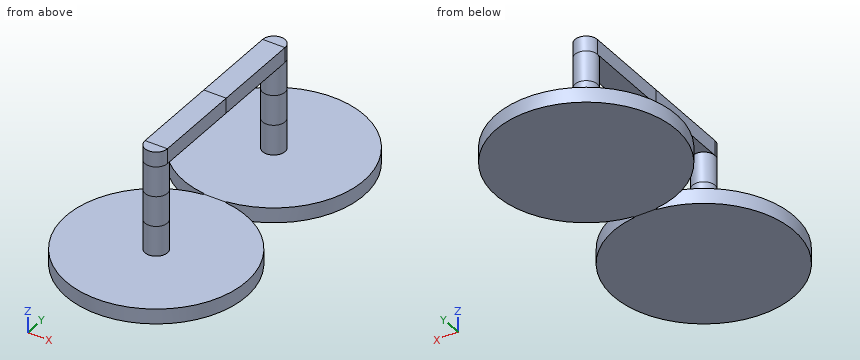
from build123d import *

# Parameters (mm, degrees)
SKETCH_1_R                       = 1.49
EXTRUDE_1_DEPTH                  = 4
EXTRUDE_START                    = 4
SKETCH_2_R                       = 1.49
EXTRUDE_2_DEPTH                  = 4
SKETCH_3_R                       = 1.49
EXTRUDE_3_DEPTH                  = 4
SKETCH_4_W                       = 2.98
SKETCH_4_H                       = 2
EXTRUDE_4_DEPTH                  = 12
EXTRUDE_4_DIRECTION_2_REACH      = 10.273
EXTRUDE_4_DIRECTION_2_END_RADIUS = 1.49
SKETCH_9_R                       = 12
EXTRUDE_6_DEPTH                  = 2
SKETCH_6_W                       = 2.98
SKETCH_6_H                       = 2
EXTRUDE_5_DEPTH                  = 12
EXTRUDE_5_DIRECTION_2_REACH      = 20.762
EXTRUDE_5_DIRECTION_2_END_RADIUS = 1.49


with BuildPart() as part:
    # 草图1 → 凸台-拉伸1 (new body)
    with BuildSketch(Plane.XY):
        Circle(SKETCH_1_R)
    extrude(amount=EXTRUDE_1_DEPTH)

    # 草图2 → 凸台-拉伸2 (add)
    with BuildSketch(Plane(origin=(0, 0, 0), x_dir=(-1, 0, 0), z_dir=(0, 0, -1)).offset(EXTRUDE_START)):
        Circle(SKETCH_2_R)
    extrude(amount=-EXTRUDE_2_DEPTH)

    # 草图3 → 凸台-拉伸3 (add)
    with BuildSketch(Plane.XY.offset(4)):
        with Locations(Location((0, 0, 0), (0, 0, 180))):
            Circle(SKETCH_3_R)
    extrude(amount=EXTRUDE_3_DEPTH)

    # 草图4 → 凸台-拉伸4 (add)
    with BuildSketch(Plane(origin=(0, 0, 0), x_dir=(1, 0, 0), z_dir=(0, 1, 0))):
        with Locations((0, 5)):
            Rectangle(SKETCH_4_W, SKETCH_4_H)
    extrude(amount=EXTRUDE_4_DEPTH)

    # 凸台-拉伸4 direction 2: up to this cylinder (the profile starts inside it)
    extrude_4_direction_2_end = Plane(origin=(0, 0, -5), z_dir=(0, 0, -1)) * Cylinder(EXTRUDE_4_DIRECTION_2_END_RADIUS, 24.526, mode=Mode.PRIVATE)
    # 草图4 → 凸台-拉伸4 direction 2 (add, up to the surface)
    with BuildSketch(Plane(origin=(0, 0, 0), x_dir=(1, 0, 0), z_dir=(0, 1, 0)), mode=Mode.PRIVATE) as extrude_4_direction_2_sk1:
        with Locations((0, 5)):
            Rectangle(SKETCH_4_W, SKETCH_4_H)
    extrude_4_direction_2_tool1 = extrude(extrude_4_direction_2_sk1.sketch, amount=-EXTRUDE_4_DIRECTION_2_REACH, mode=Mode.PRIVATE) & extrude_4_direction_2_end
    add(extrude_4_direction_2_tool1.solids().sort_by_distance((0, 0, -5))[0])

    # 草图9 → 凸台-拉伸6 (add)
    with BuildSketch(Plane(origin=(0, 0, -6), x_dir=(-1, 0, 0), z_dir=(0, 0, -1))):
        Circle(SKETCH_9_R)
    extrude(amount=-EXTRUDE_6_DEPTH)

    # 草图6 → 凸台-拉伸5 (add)
    with BuildSketch(Plane(origin=(0, 0, 0), x_dir=(1, 0, 0), z_dir=(0, 1, 0))):
        with Locations((0, -9)):
            Rectangle(SKETCH_6_W, SKETCH_6_H)
    extrude(amount=EXTRUDE_5_DEPTH)

    # 凸台-拉伸5 direction 2: up to this cylinder (the profile starts inside it)
    extrude_5_direction_2_end = Plane(origin=(0, 0, 9), z_dir=(0, 0, -1)) * Cylinder(EXTRUDE_5_DIRECTION_2_END_RADIUS, 45.504, mode=Mode.PRIVATE)
    # 草图6 → 凸台-拉伸5 direction 2 (add, up to the surface)
    with BuildSketch(Plane(origin=(0, 0, 0), x_dir=(1, 0, 0), z_dir=(0, 1, 0)), mode=Mode.PRIVATE) as extrude_5_direction_2_sk1:
        with Locations((0, -9)):
            Rectangle(SKETCH_6_W, SKETCH_6_H)
    extrude_5_direction_2_tool1 = extrude(extrude_5_direction_2_sk1.sketch, amount=-EXTRUDE_5_DIRECTION_2_REACH, mode=Mode.PRIVATE) & extrude_5_direction_2_end
    add(extrude_5_direction_2_tool1.solids().sort_by_distance((0, 0, 9))[0])

    # 镜向2: part across plane


with BuildPart() as part_1:
    add(part.part)
    add(part.part.mirror(Plane.ZX.offset(12)))


solid = part_1.part
The listing builds one solid part. Answer for the finished solid, in the listing's coordinates (mm). Coordinates: 2 decimals unless noted, no trailing zeros. Write each loop counter-clockwise with the first axis right and the second up, starting at its lowest first coordinate (ties: lowest second). Pieces come first, ordered by that corner, then holes. Notation, with made-up numbers: (19.5, 86) - (61.5, 86) arc R30 ccw to (61.5, 113) - close; hole circle Ø9 at (-11.5, 77). An arc over 180 degrees is marked (long way). Return JSON: item names as keys, results as strings.
1. The part is cut by section A-A on x = -3. Determine the outline of the cut face in (y, z).
Final values:
{"outline": "(-11.62, -6) - (11.62, -6) - (11.62, -4) - (-11.62, -4) - close; (12.38, -6) - (35.62, -6) - (35.62, -4) - (12.38, -4) - close"}
2. The part is cut by section B-B on y = 2.5. Determine the outline of the cut face in (x, z).
Final values:
{"outline": "(-11.74, -6) - (11.74, -6) - (11.74, -4) - (-11.74, -4) - close; (-1.49, 8) - (1.49, 8) - (1.49, 10) - (-1.49, 10) - close"}
3. The part is cut by section C-C on x = 0. Determine the outline of the cut face in (y, z), then the cut area to 3 significant figures.
Final values:
{"outline": "(-12, -6) - (36, -6) - (36, -4) - (25.49, -4) - (25.49, 10) - (-1.49, 10) - (-1.49, -4) - (-12, -4) - close; hole (1.49, -4) - (22.51, -4) - (22.51, 8) - (1.49, 8) - close", "area": "221 mm^2"}
4. Each of these flat-tipped pins is pushed along its axis until it touches: pin 1 Ø2 at (x, y) = (6.5, 24.5) entering from +Z; pin 2 Ø2 at (y, z) = (20.5, 9) entering from -X; pin 3 Ø0.6 at (y, z) = (15, 8.5) entering from +X. Where does it stop, or does it pass through?
Final values:
{"pin 1": "z = -4", "pin 2": "x = -1.49", "pin 3": "x = 1.49"}
5. Consider line 1 along Z through (x, y) = (-3.25, 14); line 2 along Y through (x, z) = (-7, -5); line 3 along Y through (x, z) = (-6, -4.5). Determine where each line is inside the solid, lowest interval first.
Final values:
{"line 1": "-6 to -4", "line 2": "-9.75 to 9.75, 14.25 to 33.75", "line 3": "-10.39 to 10.39, 13.61 to 34.39"}
6. The part is cut by section D-D on z = 2.5. Determine the outline of the cut face in (x, y), then the cut area to 3 significant figures.
Final values:
{"outline": "circle Ø2.98 at (0, 0); circle Ø2.98 at (0, 24)", "area": "13.9 mm^2"}
